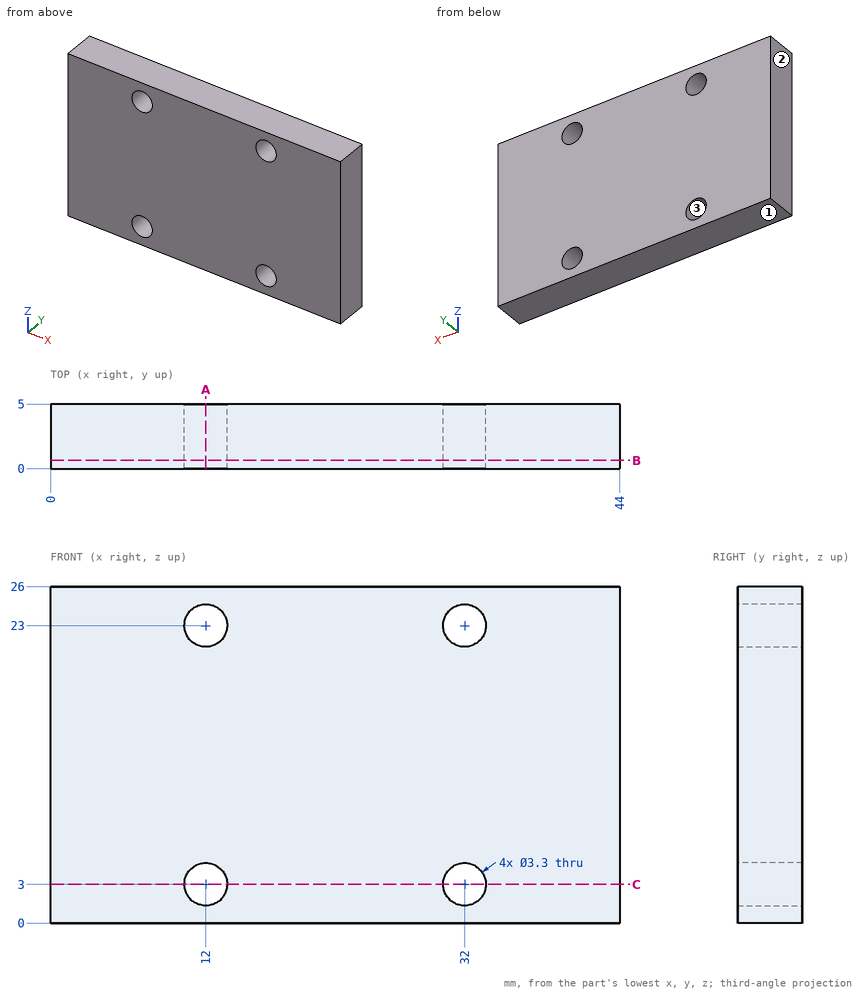
For this review, use the dimensioned drawing (mm, ordinates from the lowest corner) and the shaded views. Round coordinates to 2 decimals unless told otherwise and drop trailing zeros. Loops run counter-clockwise (first coordinate to the right, second up) from the corner with the lowest first, then second, coordinate; pieces in that order, holes last. Notation, with made-up numbers: M -24.5,-13.75 L 9.5,-13.75 A25 ccw 9.5,23.25 Z; hole C 0.25,-18 d6. An arc over 180 degrees is marked long. Answer as CSV lines item,"result".
1. To check wall thickness, follow L1, parallel to X at y = 3.8, z = 23; L2, parallel to X at y = 2.5, z = 2.25; L3, parallel to Z at x = 11, y = 2. State the ranges of each line that lie inside material, in increasing order. Write a range as [from, to].
Outcome:
L1,"x = [0, 10.35], [13.65, 30.35], [33.65, 44]"
L2,"x = [0, 10.53], [13.47, 30.53], [33.47, 44]"
L3,"z = [0, 1.69], [4.31, 21.69], [24.31, 26]"
2. We need section A-A (x = 12). Give the boundary of the cut face in (y, z), plus the area to 3 significant figures.
Outcome:
outline,"M 0,0 L 5,0 L 5,1.35 L 0,1.35 Z; M 0,4.65 L 5,4.65 L 5,21.35 L 0,21.35 Z; M 0,24.65 L 5,24.65 L 5,26 L 0,26 Z"
area,"97.0 mm2"
3. We need section B-B (y = 0.65). Give the boundary of the cut face in (x, z), plus the area to 3 significant figures.
Outcome:
outline,"M 0,0 L 44,0 L 44,26 L 0,26 Z; hole C 12,3 d3.3; hole C 12,23 d3.3; hole C 32,3 d3.3; hole C 32,23 d3.3"
area,"1,110 mm2"
4. Draft analysis for pull direction X (two halves, no side actions). For the marked faces 1, 2 and 3, state which applies: pulls with the +X half, pulls with the -X half, needs draft (parallel to the pull), parting line crosses it, or undercut.
Outcome:
face 1,"needs draft"
face 2,"pulls with the -X half"
face 3,"undercut"
5. We need section C-C (z = 3). Give the boundary of the cut face in (x, y), plus the area to 3 significant figures.
Outcome:
outline,"M 0,0 L 10.35,0 L 10.35,5 L 0,5 Z; M 13.65,0 L 30.35,0 L 30.35,5 L 13.65,5 Z; M 33.65,0 L 44,0 L 44,5 L 33.65,5 Z"
area,"187 mm2"
6. Insertion check: pin 1 Ø3 at (x, z) = (12, 3) entering from -Y. The pin has a flat end and moves straight along its axis. Give the tip position at first contact, or say it passes through.
Outcome:
pin 1,"passes through"
